The model under review builds one solid part; all positions refer to its coordinate system, in mm. A direction names the side the tool comes from. Give positions to 0.01 mm unless a question says otherwise; leave off trailing zeros. Write each loop counter-clockwise with the first axis right and the second up, starting at its lowest first coordinate (ties: lowest second). Pieces come first, ordered by that corner, then holes. Notation, with made-up numbers: (46.25, 5.5) - (56.25, 5.5) arc R12 ccw to (56.25, 25.5) - close; hole circle Ø6 at (-17, 45). An arc over 180 degrees is marked (long way). One line per question, with ' | ' between items. Start each with the question number.
```python
from build123d import *

# Parameters (mm, degrees)
CROQUIS1_R              = 10.25
CROQUIS1_R_2            = 2.5
SALIENTE_EXTRUIR1_DEPTH = 15
SALIENTE_EXTRUIR2_START = 15
CROQUIS2_R              = 10.25
CROQUIS2_R_2            = 4
SALIENTE_EXTRUIR2_DEPTH = 15


with BuildPart() as part:
    # Croquis1 → Saliente-Extruir1 (new body)
    with BuildSketch(Plane.XY):
        Circle(CROQUIS1_R)
        Circle(CROQUIS1_R_2, mode=Mode.SUBTRACT)
    extrude(amount=SALIENTE_EXTRUIR1_DEPTH)

    # Croquis2 → Saliente-Extruir2 (add)
    with BuildSketch(Plane(origin=(0, 0, 0), x_dir=(-1, 0, 0), z_dir=(0, 0, -1)).offset(SALIENTE_EXTRUIR2_START)):
        Circle(CROQUIS2_R)
        Circle(CROQUIS2_R_2, mode=Mode.SUBTRACT)
    extrude(amount=-SALIENTE_EXTRUIR2_DEPTH)


solid = part.part
```
Item 1: Take a section at A-A (x = 0). Give the boundary of the cut face in (y, z).
Item 2: Take a section at D-D (y = 6). Give the boundary of the cut face in (x, z), plus the area to 3 significant figures.
Item 3: Clearance check with flat-ended pins moving along their axes: P1, Ø7, axis at x = 0, y = 0, coming from the -Z side; P2, Ø4.5, axis at x = 0, y = 0, coming from the -Z side; P3, Ø6, axis at y = -5.5, z = 8, coming from the -X side; P4, Ø2, axis at y = -3, z = 4, coming from the +X side. State where each tip first meets the part, or that it passes through.
Item 4: Take a section at C-C (z = -8). Give the boundary of the cut face in (x, y), plus the area to 3 significant figures.
Item 5: Machinability: for faces 1 (the flat face through (-4.4, 0.1, -15)), 2 (the cylindrical face through (0.867, -3.905, -7.605)), which of the approach directions +Z, -Z, +X, -X, +Y, -Y give a long, thin tool a straight path to every point of the face, cutting with its end or side? Answer none if there is none.
Item 6: For probe 1 along Y at (x, z) = (0, 10.5); probe 2 along X at (y, z) = (-0.5, -11.75); probe 3 along Y at (x, z) = (0, -10), list the stretches that pass through material, from the lowest coordinate up.
Check sheet entries:
1) outline: (-10.25, -15) - (-4, -15) - (-4, 0) - (-2.5, 0) - (-2.5, 15) - (-10.25, 15) - close; (2.5, 0) - (4, 0) - (4, -15) - (10.25, -15) - (10.25, 15) - (2.5, 15) - close
2) outline: (-8.31, -15) - (8.31, -15) - (8.31, 15) - (-8.31, 15) - close | area: 499 mm^2
3) P1: stops at z = 0 | P2: passes through | P3: stops at x = -9.94 | P4: stops at x = 10.05
4) outline: circle Ø20.5 at (0, 0); hole circle Ø8 at (0, 0) | area: 280 mm^2
5) face 1: -Z, +X, -X, +Y, -Y | face 2: -Z
6) probe 1: y = -10.25 to -2.5, 2.5 to 10.25 | probe 2: x = -10.24 to -3.97, 3.97 to 10.24 | probe 3: y = -10.25 to -4, 4 to 10.25
